Autodesk Fusion 360 part; units mm, degrees
sketch "Sketch1" plane through (0, 0, 0) normal (0, 0, 1) x (1, 0, 0)
  circle A0 centre (0, 0) radius 2.5
  circle A1 centre (0, 0) radius 3.25
  dimension "d1" = 5
  dimension "d2" = 6.5
extrude "Extrude1" add sketch "Sketch1" along normal blind 2 contours A0 | A1
extrude "Extrude2" add sketch "Sketch1" along normal blind 11 contours A0
fillet "Fillet1" radius 0.7 1 edges at (-2.3308, -0.904, 11)
Design review of the part built by this model. Coordinates are the model's own, in mm. A direction names the side the tool comes from. Coordinates: 2 decimals unless noted, no trailing zeros. Order: outer loops, then holes, each group sorted by start corner. A loop starts at its lowest first (then second) coordinate and runs counter-clockwise, first axis right, second up.
1) Clearance check with flat-ended pins moving along their axes: pin 1 (3 mm diameter, centred on x = 1, z = 7.5, fed in from +Y); pin 2 (1 mm diameter, centred on x = 0.5, y = 2.5, fed in from +Z). State where each tip first meets the part, or that it passes through.
2) Take a section at C-C, the plane z = 1.5. Give the boundary of the cut face in (x, y), and give its area (3 significant figures).
3) Wall thickness on line 1 along Z through (x, y) = (-1.25, -2.5); line 2 along X through (y, z) = (-0.25, 10.5); line 3 along Y through (x, z) = (1.75, 7): over which ranges is each line inside the solid? List them lowest first.
4) Take a section at D-D, the plane z = 5.75. Give the boundary of the cut face in (x, y).
5) Take a section at A-A, the plane x = 0. Give the boundary of the cut face in (y, z).
6) For faces 1 (the flat face through (0, 0, 0)), 2 (the flat face through (2, -2, 2)), list the 3-axis set-ups (+Z, -Z, +X, -X, +Y, -Y) from which the entire face can be reached by the end or side of a thin tool; tool diameter is ignored.
Returned:
1. pin 1: stops at y = 2.5
1. pin 2: stops at z = 10.95
2. outline: circle Ø6.5 at (0, 0)
2. area: 33.2 mm2
3. line 1: z = 0 to 2
3. line 2: x = -2.46 to 2.46
3. line 3: y = -1.79 to 1.79
4. outline: circle Ø5 at (0, 0)
5. outline: (-3.25, 0) - (3.25, 0) - (3.25, 2) - (2.5, 2) - (2.5, 10.3) arc R0.7 ccw to (1.8, 11) - (-1.8, 11) arc R0.7 ccw to (-2.5, 10.3) - (-2.5, 2) - (-3.25, 2) - close
6. face 1: -Z, +X, -X, +Y, -Y
6. face 2: +Z
